Geometry: final body of the model. Coordinates: model frame, mm. Face numbers are marked on the shaded views. A direction names the side the tool comes from. Give positions to 0.01 mm unless a question says otherwise; leave off trailing zeros. Write each loop counter-clockwise with the first axis right and the second up, starting at its lowest first coordinate (ties: lowest second). Pieces come first, ordered by that corner, then holes.
from build123d import *

# Parameters (mm, degrees)
F1_DEPTH      = 22.352
F1_DEPTH_BACK = 22.352
F3_DEPTH      = 3.175
F3_DEPTH_BACK = 3.175
F4_R          = 10.922
F5_R          = 22.35199
F7_DEPTH      = 9.652
F9_R          = 6.35
F9_R_2        = 3.175
F10_DEPTH     = 3.175
F11_DEPTH     = 28.5637839421
F12_R         = 6.35
F12_R_2       = 3.175
F13_DEPTH     = 3.1877
F14_DEPTH     = 28.5637839421


# Not quite as in the source:
# - a fillet or chamfer is up to 0.001 mm smaller than in the source, because OpenCascade refuses the exact size


with BuildPart() as f1:
    # F0 (on Front) → F1 (new body, two sides)
    with BuildSketch(Plane.XZ) as f1_sk:
        Polygon((-21.8362923991, 37.8215678842), (0, 0), (91.4245847982, 0), (91.4245847982, 9.652), (5.5725847982, 9.652), (-13.4774152018, 42.6475678842), align=None)
    extrude(amount=F1_DEPTH)
    extrude(f1_sk.sketch, amount=-F1_DEPTH_BACK)

    # F2 (on Front) → F3 (join, two sides)
    with BuildSketch(Plane.XZ) as f3_sk:
        Polygon((30.9725847982, 9.652), (-13.4774152018, 42.6475678842), (5.5725847982, 9.652), align=None)
    extrude(amount=F3_DEPTH)
    extrude(f3_sk.sketch, amount=-F3_DEPTH_BACK)

    # F4
    f4_edges = [f1.edges().sort_by_distance(p)[0] for p in [
        (-17.656854, -22.352, 40.234568),
        (-17.656854, 22.352, 40.234568),
    ]]
    fillet(f4_edges, radius=F4_R)

    # F5 (radius 22.352 in the source; OpenCascade refuses exactly that, so slightly less here)
    f5_edges = [f1.edges().sort_by_distance(p)[0] for p in [
        (91.424585, -22.352, 4.826),
        (91.424585, 22.352, 4.826),
    ]]
    fillet(f5_edges, radius=F5_R)

    # F6 (on face) → F7 (cut, through all)
    with BuildSketch(Plane.XY.offset(9.652)):
        with BuildLine():
            Line((43.6725847982, -9.652), (69.0725847982, -9.652))
            ThreePointArc((69.0725847982, -9.652), (78.7245847982, 0), (69.0725847982, 9.652))
            Line((69.0725847982, 9.652), (43.6725847982, 9.652))
            ThreePointArc((43.6725847982, 9.652), (34.0205847982, 0), (43.6725847982, -9.652))
        make_face()
    extrude(amount=-F7_DEPTH, mode=Mode.SUBTRACT)

    # F9 (on face) → F10 (cut)
    with BuildSketch(Plane(origin=(8.3588771973, 0, 4.826), x_dir=(0, 1, 0), z_dir=(0.8660254038, 0, 0.5))):
        with Locations((-11.43, 32.7505847982)):
            Circle(F9_R)
        with Locations((-11.43, 32.7505847982)):
            Circle(F9_R_2, mode=Mode.SUBTRACT)
        with Locations((-11.43, 32.7505847982)):
            Circle(F9_R_2)
    extrude(amount=-F10_DEPTH, mode=Mode.SUBTRACT)

    # F9 (on face) → F11 (cut, through all)
    with BuildSketch(Plane(origin=(8.3588771973, 0, 4.826), x_dir=(0, 1, 0), z_dir=(0.8660254038, 0, 0.5))):
        with Locations((-11.43, 32.7505847982)):
            Circle(F9_R_2)
    extrude(amount=-F11_DEPTH, mode=Mode.SUBTRACT)

    # F12 (on face) → F13 (cut)
    with BuildSketch(Plane(origin=(8.3588771973, 0, 4.826), x_dir=(0, 1, 0), z_dir=(0.8660254038, 0, 0.5))):
        with Locations((11.43, 32.7505847982)):
            Circle(F12_R)
        with Locations((11.43, 32.7505847982)):
            Circle(F12_R_2, mode=Mode.SUBTRACT)
        with Locations((11.43, 32.7505847982)):
            Circle(F12_R_2)
    extrude(amount=-F13_DEPTH, mode=Mode.SUBTRACT)

    # F12 (on face) → F14 (cut, through all)
    with BuildSketch(Plane(origin=(8.3588771973, 0, 4.826), x_dir=(0, 1, 0), z_dir=(0.8660254038, 0, 0.5))):
        with Locations((11.43, 32.7505847982)):
            Circle(F12_R_2)
    extrude(amount=-F14_DEPTH, mode=Mode.SUBTRACT)


solid = f1.part
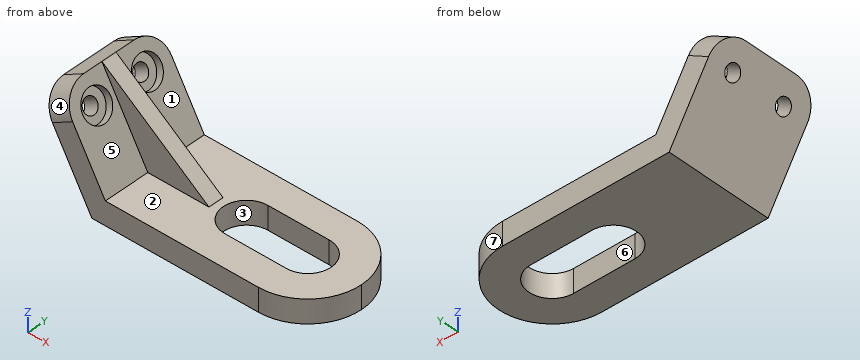
Q1. Ray query, line 1 along Y through (x, z) = (61, 8); line 2 along Z through (x, y) = (58, -12.5); line 3 along X through (y, z) = (4.5, 9). Return the intervals inside material, ascending.
Filled sheet:
line 1: y = -22.35 to -9.65, 9.65 to 22.35
line 2: z = 0 to 9.65
line 3: x = -5.2 to 35.13, 77.61 to 90.97
Q2. Pull-direction query (X, two-part tool) for the marked faces 1, 2, 3 and 4; classes: released by +X, released by -X, zero draft, split by the parting line, or undercut.
Filled sheet:
face 1: released by +X
face 2: zero draft
face 3: undercut
face 4: released by -X
Q3. Section B-B on x = 39. Output: boundary loops of the cut face in (y, z), plus the area to 3 significant figures.
Filled sheet:
outline: (-22.35, 0) - (-8.45, 0) - (-8.45, 9.65) - (-22.35, 9.65) - close; (8.45, 0) - (22.35, 0) - (22.35, 9.65) - (8.45, 9.65) - close
area: 268 mm2
Q4. Section A-A on y = 6.5. Output: boundary loops of the cut face in (x, z), plus the area to 3 significant figures.
Filled sheet:
outline: (-21.84, 37.82) - (0, 0) - (36.54, 0) - (36.54, 9.65) - (5.57, 9.65) - (-6.02, 29.72) - (-8.78, 28.13) - (-12.78, 35.06) - (-10.02, 36.65) - (-13.48, 42.65) - close; (76.21, 0) - (90.46, 0) - (90.46, 9.65) - (76.21, 9.65) - close
area: 832 mm2
Q5. Pin query (flat end, axial travel): P1, Ø3, axis at y = 13.5, z = 4.5, coming from the +X side; P2, Ø6, axis at y = -12, z = 7, coming from the +X side; P3, Ø10, axis at x = 9, z = 29, coming from the -Y side (3 decimals). Return the tip coordinate at first contact, or that it passes through.
Filled sheet:
P1: stops at x = 87.93
P2: stops at x = 89.53
P3: stops at y = -3.175
Q6. Section D-D on x = 16. Output: boundary loops of the cut face in (y, z) (3 decimals).
Filled sheet:
outline: (-22.352, 0) - (22.352, 0) - (22.352, 9.652) - (3.175, 9.652) - (3.175, 20.766) - (-3.175, 20.766) - (-3.175, 9.652) - (-22.352, 9.652) - close
Q7. Access query for the marked faces 5, 6 and 7. Directions: +Z, -Z, +X, -X, +Y, -Y. A direction counts if a zero-diameter tool reaches every point of the face in a straight line with its end or side. Return the directions, or none.
Filled sheet:
face 5: +Z, +X, -Y
face 6: +Z, -Z
face 7: +Z, -Z, +X, +Y
